Read the model definition and answer for the solid it produces. Units are mm, in the model's axes. Coordinates: 2 decimals unless noted, no trailing zeros. Order: outer loops, then holes, each group sorted by start corner. A loop starts at its lowest first (then second) coordinate and runs counter-clockwise, first axis right, second up. Notation, with made-up numbers: (68, -38) - (91, -38) arc R28 cw to (91, -6) - close; hole circle Ø7 at (58, 18). An arc over 180 degrees is marked (long way). Write item = value, one per line.
from build123d import *

# Parameters (mm, degrees)
SKETCH1_R           = 2.5
BOSS_EXTRUDE1_DEPTH = 9
SKETCH2_W           = 1.5
SKETCH2_H           = 71.396737885
CUT_EXTRUDE1_DEPTH  = 10
BOSS_EXTRUDE2_DEPTH = 70.368354
FILLET1_R           = 0.5
FILLET2_R           = 5


with BuildPart() as part:
    # Sketch1 → Boss-Extrude1 (new body)
    with BuildSketch(Plane.XY):
        with BuildLine():
            Line((-11.03377919, 0), (-30.129933814, -40.951835747))
            ThreePointArc((-30.129933814, -40.951835747), (-27.711486187, -47.596465991), (-21.066855944, -45.178018364))
            Line((-21.066855944, -45.178018364), (0, 0))
            ThreePointArc((0, 0), (5.707925077, 13.632041213), (15.151572114, 25))
            Line((15.151572114, 25), (15.151572114, 95))
            ThreePointArc((15.151572114, 95), (7.05920736, 86.420861211), (4.117792925, 75))
            Line((4.117792925, 75), (4.117792925, 25))
            ThreePointArc((4.117792925, 25), (-5.106750503, 13.499250648), (-11.03377919, 0))
        make_face()
        with Locations((-25.598394879, -43.064927056)):
            Circle(SKETCH1_R, mode=Mode.SUBTRACT)
        with Locations((-7.848427886, -5)):
            Circle(SKETCH1_R, mode=Mode.SUBTRACT)
    extrude(amount=BOSS_EXTRUDE1_DEPTH)

    # Sketch2 → Cut-Extrude1 (cut, through all)
    with BuildSketch(Plane.XY.offset(9)):
        with Locations((14.401572114, 59.301631058)):
            Rectangle(SKETCH2_W, SKETCH2_H)
    extrude(amount=-CUT_EXTRUDE1_DEPTH, mode=Mode.SUBTRACT)

    # Sketch4 → Boss-Extrude2 (add)
    with BuildSketch(Plane(origin=(0, 93.971615681, 0), x_dir=(0, 0, -1), z_dir=(0, -1, 0))):
        Polygon((0, 13.651572114), (-4.5, 16.249648326), (-9, 13.651572114), align=None)
    extrude(amount=BOSS_EXTRUDE2_DEPTH)

    # Fillet1
    fillet1_edges = [part.edges().sort_by_distance(p)[0] for p in [
        (16.249648326, 58.787438681, 4.5),
    ]]
    fillet(fillet1_edges, radius=FILLET1_R)

    # Fillet2
    fillet2_edges = [part.edges().sort_by_distance(p)[0] for p in [
        (0, 0, 4.5),
        (-11.03377919, 0, 4.5),
        (4.117792925, 25, 4.5),
        (13.651572114, 23.603262115, 4.5),
    ]]
    fillet(fillet2_edges, radius=FILLET2_R)


solid = part.part
1) Straight lines are drawn through the part: line 1 along X through (y, z) = (-41.5, 2.5); line 2 along Y through (x, z) = (-8, 1.75); line 3 along X through (y, z) = (26.5, 2.75). For each, find the intervals that lie inside material, in ascending order. Write a range as from..to.
Returned:
line_1 = -30.35..-27.55, -23.65..-19.35
line_2 = -17.16..-7.5, -2.5..8.08
line_3 = 4.08..15.24
2) The part is cut by section A-A (z = 1.5). Determine the outline of the cut face in (x, y), and give its area (3 significant figures).
Returned:
outline = (-30.13, -40.95) arc R5 ccw to (-21.07, -45.18) - (-0.19, -0.42) arc R5 ccw to (0.11, 0.43) arc R50 cw to (12.1, 22.04) arc R5 cw to (14.52, 23.45) - (14.52, 93.97) - (13.65, 93.97) arc R23.64 ccw to (4.12, 75) - (4.12, 27.08) arc R5 cw to (2.7, 23.59) arc R56.37 ccw to (-10.93, 0.35) arc R5 cw to (-11.19, -0.34) - close; hole circle Ø5 at (-25.6, -43.06); hole circle Ø5 at (-7.85, -5)
area = 1,410 mm^2
3) The part is cut by section D-D (x = -17). Determine the outline of the cut face in (y, z), and give its area (3 significant figures).
Returned:
outline = (-36.46, 0) - (-12.79, 0) - (-12.79, 9) - (-36.46, 9) - close
area = 213 mm^2
4) Flat-ended cylindrical pins translate along their axes: pin 1 Ø1 at (x, z) = (8, 8) entering from +Y; pin 2 Ø5 at (x, z) = (-22.5, 4.5) entering from +Y; pin 3 Ø4 at (y, z) = (13, 4.5) entering from -X; pin 4 Ø4 at (x, y) = (-25.6, -43.06) entering from -Z. Find the tip coordinate at first contact, or state that the pin passes through.
Returned:
pin_1 = 88.71
pin_2 = -19.23
pin_3 = -6.54
pin_4 = through
5) Determine the mould class of faces 1 (the face through (13.38, 23.01, 4.44)), 2 (the face through (-9.69, -3.31, 4.44)), 3 (the face through (4.118, 51, 4)) for opening direction Y: pulls with the +Y half, pulls with the -Y half, needs draft (parallel to the pull), parting line crosses it, or undercut.
Returned:
face_1 = pulls with the -Y half
face_2 = undercut
face_3 = needs draft
6) The part is cut by section B-B (y = 29.5). Determine the outline of the cut face in (x, z).
Returned:
outline = (4.12, 0) - (13.65, 0) - (16.11, 4.25) arc R0.5 ccw to (16.11, 4.75) - (13.65, 9) - (4.12, 9) - close
7) The part is cut by section C-C (y = -5). Determine the outline of the cut face in (x, z).
Returned:
outline = (-13.37, 0) - (-10.35, 0) - (-10.35, 9) - (-13.37, 9) - close; (-5.35, 0) - (-2.33, 0) - (-2.33, 9) - (-5.35, 9) - close
